Read the model definition and answer for the solid it produces. Units are mm, in the model's axes. Face numbers are marked on the shaded views. A direction names the side the tool comes from. Coordinates: 2 decimals unless noted, no trailing zeros. Order: outer loops, then holes, each group sorted by start corner. A loop starts at its lowest first (then second) coordinate and runs counter-clockwise, first axis right, second up. Notation, with made-up numbers: (30, -37) - (89, -37) arc R25 ccw to (89, -11) - close; hole circle Ø1 at (-4, -8). An arc over 180 degrees is marked (long way). Answer as a JSON object with one key per item and string values. Group by question number.
from build123d import *

# Parameters (mm, degrees)
BOSS_EXTRUDE1_DEPTH = 6
CUT_EXTRUDE1_DEPTH  = 6


with BuildPart() as part:
    # Sketch1 → Boss-Extrude1 (new body)
    with BuildSketch(Plane.XY):
        with BuildLine():
            ThreePointArc((-23.297478626, 3.98388923), (-21.550990273, 2.825758414), (-19.579218077, 2.11610853))
            ThreePointArc((-19.579218077, 2.11610853), (-19.647653189, 1.299796091), (-19.682068786, 0.481343326))
            ThreePointArc((-19.682068786, 0.481343326), (-21.727235684, 0.024417829), (-23.605104735, -0.905687747))
            ThreePointArc((-23.605104735, -0.905687747), (-23.578381459, -1.419755495), (-23.540464241, -1.93311898))
            ThreePointArc((-23.540464241, -1.93311898), (-21.560829609, -2.620530995), (-19.474521512, -2.817526118))
            ThreePointArc((-19.474521512, -2.817526118), (-19.337797961, -3.625211721), (-19.167591403, -4.426510099))
            ThreePointArc((-19.167591403, -4.426510099), (-21.034872872, -5.377692766), (-22.622437362, -6.745584408))
            ThreePointArc((-22.622437362, -6.745584408), (-22.468710197, -7.236855963), (-22.304315911, -7.724661561))
            ThreePointArc((-22.304315911, -7.724661561), (-20.215922725, -7.898162151), (-18.146169139, -7.570124585))
            ThreePointArc((-18.146169139, -7.570124585), (-17.812877768, -8.318433495), (-17.448743759, -9.052228961))
            ThreePointArc((-17.448743759, -9.052228961), (-19.020811637, -10.437902494), (-20.218319051, -12.157630537))
            ThreePointArc((-20.218319051, -12.157630537), (-19.94724724, -12.595237503), (-19.666705383, -13.026834594))
            ThreePointArc((-19.666705383, -13.026834594), (-17.600775067, -12.675522078), (-15.677626222, -11.843063629))
            ThreePointArc((-15.677626222, -11.843063629), (-15.168708954, -12.484976846), (-14.633527372, -13.105162332))
            ThreePointArc((-14.633527372, -13.105162332), (-15.811602852, -14.838259766), (-16.543809396, -16.801767375))
            ThreePointArc((-16.543809396, -16.801767375), (-16.172425378, -17.158213294), (-15.793363427, -17.506483047))
            ThreePointArc((-15.793363427, -17.506483047), (-13.879705981, -16.652431682), (-12.22400039, -15.367858777))
            ThreePointArc((-12.22400039, -15.367858777), (-11.571434369, -15.863042531), (-10.898832642, -16.330649503))
            ThreePointArc((-10.898832642, -16.330649503), (-11.60889291, -18.302273952), (-11.829791353, -20.386186721))
            ThreePointArc((-11.829791353, -20.386186721), (-11.381430551, -20.639074787), (-10.927666363, -20.882134132))
            ThreePointArc((-10.927666363, -20.882134132), (-9.286523922, -19.579007107), (-8.002295658, -17.923034185))
            ThreePointArc((-8.002295658, -17.923034185), (-7.247084006, -18.240374261), (-6.479324175, -18.526021252))
            ThreePointArc((-6.479324175, -18.526021252), (-6.676753531, -20.612288301), (-6.372464012, -22.685666328))
            ThreePointArc((-6.372464012, -22.685666328), (-5.875298584, -22.819106653), (-5.375343832, -22.941683276))
            ThreePointArc((-5.375343832, -22.941683276), (-4.109835412, -21.271360855), (-3.277777259, -19.348038785))
            ThreePointArc((-3.277777259, -19.348038785), (-2.467372703, -19.467595539), (-1.65269594, -19.553334298))
            ThreePointArc((-1.65269594, -19.553334298), (-1.325089173, -21.623156117), (-0.514731321, -23.555721434))
            ThreePointArc((-0.514731321, -23.555721434), (0, -23.561329471), (0.514731321, -23.555721434))
            ThreePointArc((0.514731321, -23.555721434), (1.325089173, -21.623156117), (1.65269594, -19.553334298))
            ThreePointArc((1.65269594, -19.553334298), (2.467372703, -19.467595539), (3.277777259, -19.348038785))
            ThreePointArc((3.277777259, -19.348038785), (4.109835412, -21.271360855), (5.375343832, -22.941683276))
            ThreePointArc((5.375343832, -22.941683276), (5.875298584, -22.819106653), (6.372464012, -22.685666328))
            ThreePointArc((6.372464012, -22.685666328), (6.676753531, -20.612288301), (6.479324175, -18.526021252))
            ThreePointArc((6.479324175, -18.526021252), (7.247084006, -18.240374261), (8.002295658, -17.923034185))
            ThreePointArc((8.002295658, -17.923034185), (9.286523922, -19.579007107), (10.927666363, -20.882134132))
            ThreePointArc((10.927666363, -20.882134132), (11.381430551, -20.639074787), (11.829791353, -20.386186721))
            ThreePointArc((11.829791353, -20.386186721), (11.60889291, -18.302273952), (10.898832642, -16.330649503))
            ThreePointArc((10.898832642, -16.330649503), (11.571434369, -15.863042531), (12.22400039, -15.367858777))
            ThreePointArc((12.22400039, -15.367858777), (13.879705981, -16.652431682), (15.793363427, -17.506483047))
            ThreePointArc((15.793363427, -17.506483047), (16.172425378, -17.158213294), (16.543809396, -16.801767375))
            ThreePointArc((16.543809396, -16.801767375), (15.811602852, -14.838259766), (14.633527372, -13.105162332))
            ThreePointArc((14.633527372, -13.105162332), (15.168708954, -12.484976846), (15.677626222, -11.843063629))
            ThreePointArc((15.677626222, -11.843063629), (17.600775067, -12.675522078), (19.666705383, -13.026834594))
            ThreePointArc((19.666705383, -13.026834594), (19.94724724, -12.595237503), (20.218319051, -12.157630537))
            ThreePointArc((20.218319051, -12.157630537), (19.020811637, -10.437902494), (17.448743759, -9.052228961))
            ThreePointArc((17.448743759, -9.052228961), (17.812877768, -8.318433495), (18.146169139, -7.570124585))
            ThreePointArc((18.146169139, -7.570124585), (20.215922725, -7.898162151), (22.304315911, -7.724661561))
            ThreePointArc((22.304315911, -7.724661561), (22.468710197, -7.236855963), (22.622437362, -6.745584408))
            ThreePointArc((22.622437362, -6.745584408), (21.034872872, -5.377692766), (19.167591403, -4.426510099))
            ThreePointArc((19.167591403, -4.426510099), (19.337797961, -3.625211721), (19.474521512, -2.817526118))
            ThreePointArc((19.474521512, -2.817526118), (21.560829609, -2.620530995), (23.540464241, -1.93311898))
            ThreePointArc((23.540464241, -1.93311898), (23.578381459, -1.419755495), (23.605104735, -0.905687747))
            ThreePointArc((23.605104735, -0.905687747), (21.727235684, 0.024417829), (19.682068786, 0.481343326))
            ThreePointArc((19.682068786, 0.481343326), (19.647653189, 1.299796091), (19.579218077, 2.11610853))
            ThreePointArc((19.579218077, 2.11610853), (21.550990273, 2.825758414), (23.297478626, 3.98388923))
            ThreePointArc((23.297478626, 3.98388923), (23.206536298, 4.490554086), (23.104576563, 4.995117258))
            ThreePointArc((23.104576563, 4.995117258), (21.054396371, 5.428994815), (18.959849401, 5.362952832))
            ThreePointArc((18.959849401, 5.362952832), (18.722974108, 6.147133588), (18.453680362, 6.920780951))
            ThreePointArc((18.453680362, 6.920780951), (20.18702296, 8.098495683), (21.590626747, 9.654575682))
            ThreePointArc((21.590626747, 9.654575682), (21.376539115, 10.122706292), (21.152302873, 10.586061329))
            ThreePointArc((21.152302873, 10.586061329), (19.058631901, 10.496448744), (17.046312949, 9.911588942))
            ThreePointArc((17.046312949, 9.911588942), (16.621861705, 10.612224728), (16.168630043, 11.294595904))
            ThreePointArc((16.168630043, 11.294595904), (17.554630751, 12.866375338), (18.527156386, 14.722630289))
            ThreePointArc((18.527156386, 14.722630289), (18.203375361, 15.122812286), (17.870952201, 15.515844888))
            ThreePointArc((17.870952201, 15.515844888), (15.865343497, 14.908372849), (14.061693963, 13.84144412))
            ThreePointArc((14.061693963, 13.84144412), (13.476336601, 14.414511412), (12.867645233, 14.962730512))
            ThreePointArc((12.867645233, 14.962730512), (13.819216531, 16.829813965), (14.29955665, 18.869608544))
            ThreePointArc((14.29955665, 18.869608544), (13.886426585, 19.176697021), (13.466703877, 19.474711502))
            ThreePointArc((13.466703877, 19.474711502), (11.675177211, 18.387549712), (10.19352703, 16.905591112))
            ThreePointArc((10.19352703, 16.905591112), (9.484043705, 17.315081985), (8.75813895, 17.694702387))
            ThreePointArc((8.75813895, 17.694702387), (9.215490113, 19.739774138), (9.17346318, 21.834940549))
            ThreePointArc((9.17346318, 21.834940549), (8.696942557, 22.029640008), (8.216293022, 22.213911023))
            ThreePointArc((8.216293022, 22.213911023), (6.751416603, 20.715369856), (5.684863304, 18.911498294))
            ThreePointArc((5.684863304, 18.911498294), (4.895833464, 19.13168293), (4.098326587, 19.318851687))
            ThreePointArc((4.098326587, 19.318851687), (4.032720558, 21.413412357), (3.47096728, 23.43230359))
            ThreePointArc((3.47096728, 23.43230359), (2.960997643, 23.502380347), (2.449622259, 23.561329471))
            ThreePointArc((2.449622259, 23.561329471), (1.40343966, 21.745567779), (0.818998709, 19.733127139))
            ThreePointArc((0.818998709, 19.733127139), (0, 19.750170529), (-0.818998709, 19.733127139))
            ThreePointArc((-0.818998709, 19.733127139), (-1.40343966, 21.745567779), (-2.449622259, 23.561329471))
            ThreePointArc((-2.449622259, 23.561329471), (-2.960997643, 23.502380347), (-3.47096728, 23.43230359))
            ThreePointArc((-3.47096728, 23.43230359), (-4.032720558, 21.413412357), (-4.098326587, 19.318851687))
            ThreePointArc((-4.098326587, 19.318851687), (-4.895833464, 19.13168293), (-5.684863304, 18.911498294))
            ThreePointArc((-5.684863304, 18.911498294), (-6.751416603, 20.715369856), (-8.216293022, 22.213911023))
            ThreePointArc((-8.216293022, 22.213911023), (-8.696942557, 22.029640008), (-9.17346318, 21.834940549))
            ThreePointArc((-9.17346318, 21.834940549), (-9.215490113, 19.739774138), (-8.75813895, 17.694702387))
            ThreePointArc((-8.75813895, 17.694702387), (-9.484043705, 17.315081985), (-10.19352703, 16.905591112))
            ThreePointArc((-10.19352703, 16.905591112), (-11.675177211, 18.387549712), (-13.466703877, 19.474711502))
            ThreePointArc((-13.466703877, 19.474711502), (-13.886426585, 19.176697021), (-14.29955665, 18.869608544))
            ThreePointArc((-14.29955665, 18.869608544), (-13.819216531, 16.829813965), (-12.867645233, 14.962730512))
            ThreePointArc((-12.867645233, 14.962730512), (-13.476336601, 14.414511412), (-14.061693963, 13.84144412))
            ThreePointArc((-14.061693963, 13.84144412), (-15.865343497, 14.908372849), (-17.870952201, 15.515844888))
            ThreePointArc((-17.870952201, 15.515844888), (-18.203375361, 15.122812286), (-18.527156386, 14.722630289))
            ThreePointArc((-18.527156386, 14.722630289), (-17.554630751, 12.866375338), (-16.168630043, 11.294595904))
            ThreePointArc((-16.168630043, 11.294595904), (-16.621861705, 10.612224728), (-17.046312949, 9.911588942))
            ThreePointArc((-17.046312949, 9.911588942), (-19.058631901, 10.496448744), (-21.152302873, 10.586061329))
            ThreePointArc((-21.152302873, 10.586061329), (-21.376539115, 10.122706292), (-21.590626747, 9.654575682))
            ThreePointArc((-21.590626747, 9.654575682), (-20.18702296, 8.098495683), (-18.453680362, 6.920780951))
            ThreePointArc((-18.453680362, 6.920780951), (-18.722974108, 6.147133588), (-18.959849401, 5.362952832))
            ThreePointArc((-18.959849401, 5.362952832), (-21.054396371, 5.428994815), (-23.104576563, 4.995117258))
            ThreePointArc((-23.104576563, 4.995117258), (-23.206536298, 4.490554086), (-23.297478626, 3.98388923))
        make_face()
    extrude(amount=BOSS_EXTRUDE1_DEPTH)

    # Sketch2 → Cut-Extrude1 (cut)
    with BuildSketch(Plane.XY.offset(6)):
        with BuildLine():
            Line((-1.68792147, 1.136480442), (1.106353759, 1.729798183))
            ThreePointArc((1.106353759, 1.729798183), (0.415405508, -1.892713448), (-1.68792147, 1.136480442))
        make_face()
    extrude(amount=-CUT_EXTRUDE1_DEPTH, mode=Mode.SUBTRACT)


solid = part.part
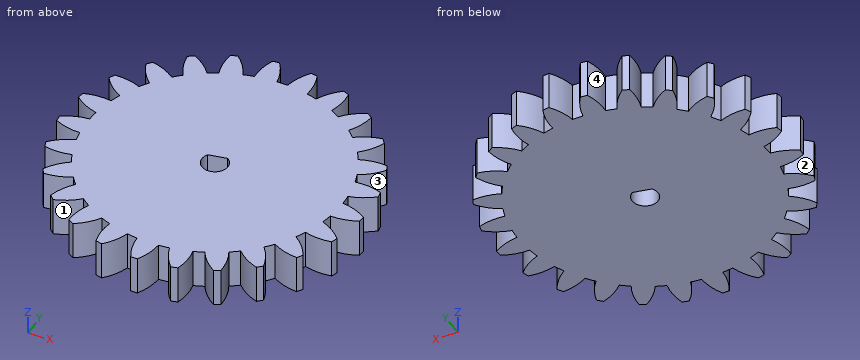
1. Given pin 1 (1 mm diameter, centred on y = -16.5, z = 2, fed in from -X), flat-ended and moving along its own axis, determine where the tip first touches the part or whether it passes through.
2. For the marked faces 1, 2, 3 and 4, determine the directions among +Z, -Z, +X, -X, +Y, -Y from which every point of the face is accessible in a straight line to the end or side of a thin tool.
3. A cutting plane is placed at A-A on y = -14.5. Write down the section's boundary in (x, z).
4. Straight lines are drawn through the part: L1, parallel to Y at x = 21, z = 4.7; L2, parallel to Y at x = 0, z = 4; L3, parallel to Y at x = -4.5, z = 3.6. For each, find the intervals that lie inside material, in ascending order.
5. A cutting plane is placed at B-B on y = 13. Write down the section's boundary in (x, z), and give its area (3 significant figures).
Derived:
{
 "1": {"pin 1": "stops at x = -16.54"},
 "2": {"face 1": "+Z, -Z, -Y", "face 2": "+Z, -Z, -X", "face 3": "+Z, -Z, +X", "face 4": "+Z, -Z"},
 "3": {"outline": "(-15.63, 0) - (15.63, 0) - (15.63, 6) - (-15.63, 6) - close"},
 "4": {"L1": "y = -7.89 to -5.35, -2.72 to 0.25, 2.57 to 5.43, 8.91 to 10.6", "L2": "y = -23.56 to -1.94, 1.49 to 19.75", "L3": "y = -21.88 to 19.23"},
 "5": {"outline": "(-17.64, 0) - (17.64, 0) - (17.64, 6) - (-17.64, 6) - close", "area": "212 mm2"}
}
